The listing builds one solid part. Answer for the finished solid, in the listing's coordinates (mm). A direction names the side the tool comes from. Round coordinates to 2 decimals unless told otherwise and drop trailing zeros. Write each loop counter-clockwise with the first axis right and the second up, starting at its lowest first coordinate (ties: lowest second). Pieces come first, ordered by that corner, then holes. Notation, with made-up numbers: (27.5, 21) - (53.5, 21) arc R19 cw to (53.5, 35) - close; hole circle Ø8 at (-15.75, -18). An arc over 180 degrees is marked (long way). Return JSON: item names as keys, results as strings. Group by question number.
(1) Section D-D, the plane z = -10 is taken. Write down the section's boundary in (x, y).
(2) Which of the six approach directions +Z, -Z, +X, -X, +Y, -Y give full straight-line access (tool end or side, diameter ignored) to faces 1 (the cylindrical face through (3.01, 12.07, 0.65)), 2 (the cylindrical face through (0.99, 16.01, 1.11))?
(3) Each of these flat-tipped pins is pushed along its axis until it touches: pin 1 (4 mm diameter, centred on y = 0, z = 0, fed in from +X); pin 2 (1 mm diameter, centred on x = 1.5, z = -9, fed in from +Y); pin 3 (1 mm diameter, centred on x = 3.5, z = -12.5, fed in from -Y). Where does it stop, or does it pass through?
(4) Section C-C, the plane x = 3.5 is taken. Write down the section's boundary in (y, z).
(5) Find the intervals of material crossed by line 1 along Y through (x, z) = (1, 0); line 2 along Y through (x, z) = (2.85, 0); line 3 along X through (y, z) = (11.25, -5.25), in increasing order. Write a range as [from, to].
(6) Section B-B, the plane z = 0 is taken. Write down the section's boundary in (x, y), then the cut area to 3 significant figures.
(7) Determine the mould class of faces 3 (the cylindrical face through (0.99, 0.07, 1.5)), 4 (the flat face through (1.972, 15.008, -7.477)), 5 (the flat face through (2, 8, 4)), 6 (the flat face through (0, 8, -3)) for opening direction Z: +Z half, -Z half, draft (parallel to the pull), parting line (faces both ways), or undercut.
(8) Section A-A, the plane y = 7.5 is taken. Write down the section's boundary in (x, z).
```python
from build123d import *
from build123d.topology import SkipClean

# Parameters (mm, degrees)
SKETCH_1_R          = 1.5
SKETCH_1_R_2        = 2.1
EXTRUDE_1_DEPTH     = 6
SKETCH_2_R          = 3
CUT_EXTRUDE_1_DEPTH = 3
SKETCH_3_R          = 3
CUT_EXTRUDE_2_DEPTH = 1
CUT_EXTRUDE_START   = -2
SKETCH_4_R          = 3
CUT_EXTRUDE_3_DEPTH = 2


with BuildPart() as part:
    # 草图1 → 凸台-拉伸1 (new body)
    with BuildSketch(Plane(origin=(0, 0, 0), x_dir=(0, 0, -1), z_dir=(1, 0, 0))):
        with BuildLine():
            Line((-4, 15), (-4, 0))
            ThreePointArc((-4, 0), (-1.930643586, -3.503229274), (2.136307673, -3.381743563))
            Line((2.136307673, -3.381743563), (12.670384591, 3.272820546))
            ThreePointArc((12.670384591, 3.272820546), (15, 7.5), (12.670384591, 11.727179454))
            Line((12.670384591, 11.727179454), (2.136307673, 18.381743563))
            ThreePointArc((2.136307673, 18.381743563), (-1.930643586, 18.503229274), (-4, 15))
        make_face()
        Circle(SKETCH_1_R, mode=Mode.SUBTRACT)
        with Locations((0, 15)):
            Circle(SKETCH_1_R, mode=Mode.SUBTRACT)
        with Locations((10, 7.5)):
            Circle(SKETCH_1_R_2, mode=Mode.SUBTRACT)
    extrude(amount=EXTRUDE_1_DEPTH)

    # 草图2 → 切除-拉伸1 (cut)
    with BuildSketch(Plane(origin=(6, 0, 0), x_dir=(0, 0, -1), z_dir=(1, 0, 0))):
        with Locations((0, 15)):
            Circle(SKETCH_2_R)
        Circle(SKETCH_2_R)
    extrude(amount=-CUT_EXTRUDE_1_DEPTH, mode=Mode.SUBTRACT)

    # 草图3 → 切除-拉伸2 (cut)
    with BuildSketch(Plane(origin=(3, 0, 0), x_dir=(0, 0, -1), z_dir=(1, 0, 0))):
        Circle(SKETCH_3_R)
        with Locations((0, 15)):
            Circle(SKETCH_3_R)
    extrude(amount=-CUT_EXTRUDE_2_DEPTH, mode=Mode.SUBTRACT)

    # 草图4 → 切除-拉伸3 (cut)
    with SkipClean():  # the faces are left unmerged after this step: merging them gives an invalid solid
        with BuildSketch(Plane(origin=(6, 0, 0), x_dir=(0, 0, -1), z_dir=(1, 0, 0)).offset(CUT_EXTRUDE_START)):
            with BuildLine():
                ThreePointArc((12.670384591, 3.272820546), (5, 7.5), (12.670384591, 11.727179454))
                Line((12.670384591, 11.727179454), (2.136307673, 18.381743563))
                ThreePointArc((2.136307673, 18.381743563), (-1.930643586, 18.503229274), (-4, 15))
                Line((-4, 15), (-4, 0))
                ThreePointArc((-4, 0), (-1.930643586, -3.503229274), (2.136307673, -3.381743563))
                Line((2.136307673, -3.381743563), (12.670384591, 3.272820546))
            make_face()
            Circle(SKETCH_4_R, mode=Mode.SUBTRACT)
            with Locations((0, 15)):
                Circle(SKETCH_4_R, mode=Mode.SUBTRACT)
        extrude(amount=CUT_EXTRUDE_3_DEPTH, mode=Mode.SUBTRACT)


solid = part.part
```
Working result:
{
 "1": {"outline": "(0, 1.59) - (4, 1.59) - (4, 2.5) - (6, 2.5) - (6, 5.4) - (0, 5.4) - close; (0, 9.6) - (6, 9.6) - (6, 12.5) - (4, 12.5) - (4, 13.41) - (0, 13.41) - close"},
 "2": {"face 1": "+X", "face 2": "+X, -X"},
 "3": {"pin 1": "stops at x = 2", "pin 2": "stops at y = 14.36", "pin 3": "stops at y = 2.85"},
 "4": {"outline": "(-3.38, -2.14) - (3.27, -12.67) arc R5 ccw to (11.73, -12.67) - (18.38, -2.14) arc R4 ccw to (15, 4) - (0, 4) arc R4 ccw to start; hole circle Ø6 at (0, 0); hole circle Ø4.2 at (7.5, -10); hole circle Ø6 at (15, 0)"},
 "5": {"line 1": "y = [-4, -1.5], [1.5, 13.5], [16.5, 19]", "line 2": "y = [-4, -3], [3, 12], [18, 19]", "line 3": "x = [0, 4]"},
 "6": {"outline": "(0, -4) - (4, -4) - (4, -3) - (2, -3) - (2, -1.5) - (0, -1.5) - close; (0, 1.5) - (2, 1.5) - (2, 3) - (4, 3) - (4, 12) - (2, 12) - (2, 13.5) - (0, 13.5) - close; (0, 16.5) - (2, 16.5) - (2, 18) - (4, 18) - (4, 19) - (0, 19) - close", "area": "56.0 mm^2"},
 "7": {"face 3": "undercut", "face 4": "-Z half", "face 5": "+Z half", "face 6": "draft"},
 "8": {"outline": "(0, -15) - (6, -15) - (6, -12.1) - (0, -12.1) - close; (0, -7.9) - (6, -7.9) - (6, -5) - (4, -5) - (4, 4) - (0, 4) - close"}
}
